```python
from build123d import *

# Parameters (mm, degrees)
ESQUISSE2_R             = 1.55
BOSS_EXTRU_1_DEPTH      = 6
ESQUISSE3_W             = 170
ESQUISSE3_H             = 35
ENL_V_MAT_EXTRU_1_DEPTH = 10
ENL_V_MAT_EXTRU_2_DEPTH = 2


with BuildPart() as part:
    # Esquisse2 → Boss.-Extru.1 (new body)
    with BuildSketch(Plane(origin=(0, 0, 0), x_dir=(1, 0, 0), z_dir=(0, 1, 0))):
        Polygon((30, 7.5), (-90, 7.5), (-100, 7.5), (-100, -7.5), (-90, -7.5), (30, -7.5), (40, -7.5), (50, -7.5), (50, 7.5), (40, 7.5), align=None)
        with Locations(Location((-90, 0, 0), (0, 0, 270))):
            Circle(ESQUISSE2_R, mode=Mode.SUBTRACT)
        with Locations(Location((0, 0, 0), (0, 0, 270))):
            Circle(ESQUISSE2_R, mode=Mode.SUBTRACT)
        with Locations(Location((40, 0, 0), (0, 0, 270))):
            Circle(ESQUISSE2_R, mode=Mode.SUBTRACT)
    extrude(amount=BOSS_EXTRU_1_DEPTH)

    # Esquisse3 → Enlèv. mat.-Extru.1 (cut)
    with BuildSketch(Plane.XZ):
        with Locations((-25, 0)):
            Rectangle(ESQUISSE3_W, ESQUISSE3_H)
        with BuildLine():
            Line((-90, -7.5), (-83.140864445, -7.5))
            Line((-83.140864445, -7.5), (-80, -5))
            Line((-80, -5), (0, -5))
            Line((0, -5), (30, -5))
            Line((30, -5), (33.140864445, -7.5))
            Line((33.140864445, -7.5), (40, -7.5))
            add(Edge.make_bspline(
                [(40, -7.5), (44.292893219, -7.707106781), (50.707106781, 0), (44.292893219, 7.707106781), (40, 7.5)],
                knots=[0, 0, 0, 0, 0.5, 1, 1, 1, 1], degree=3))
            Line((40, 7.5), (33.140864445, 7.5))
            Line((33.140864445, 7.5), (30, 5))
            Line((30, 5), (0, 5))
            Line((0, 5), (-80, 5))
            Line((-80, 5), (-83.140864445, 7.5))
            Line((-83.140864445, 7.5), (-90, 7.5))
            add(Edge.make_bspline(
                [(-90, -7.5), (-94.266151252, -7.718988485), (-100.733567708, 6.0631e-05), (-94.266713321, 7.718514748), (-90, 7.5)],
                knots=[0, 0, 0, 0, 0.500005708, 1, 1, 1, 1], degree=3))
        make_face(mode=Mode.SUBTRACT)
    extrude(amount=-ENL_V_MAT_EXTRU_1_DEPTH, mode=Mode.SUBTRACT)

    # Esquisse4 → Enlèv. mat.-Extru.2 (cut)
    with BuildSketch(Plane(origin=(0, 6, 0), x_dir=(1, 0, 0), z_dir=(0, 1, 0))):
        Polygon((-81.8, 3), (-80.7, 0), (-81.8, -3), (-8.2, -3), (-9.3, 0), (-8.2, 3), align=None)
    extrude(amount=-ENL_V_MAT_EXTRU_2_DEPTH, mode=Mode.SUBTRACT)


solid = part.part
```
Check sheet for the modelled part. Datum: model origin and axes. Units: mm. A direction names the side the tool comes from. Round coordinates to 2 decimals unless told otherwise and drop trailing zeros. Order: outer loops, then holes, each group sorted by start corner. A loop starts at its lowest first (then second) coordinate and runs counter-clockwise, first axis right, second up. Notation, with made-up numbers: (-33, 34.5) -> (23, 34.5) arc R13 ccw to (23, 41.5) -> close; hole circle Ø1 at (76, 67.25). An arc over 180 degrees is marked (long way). One line per item, written item: value. Start each with the question number.
Q1. Cross-section at A-A (x = 0). Record the boundary of the cut face in (y, z), and give its area (3 significant figures).
Q2. Mould release check, pull along X, two halves, no side actions. Record for faces 1 (the face through (-81.548, 2.958, 6.232)), 2 (the face through (-87, 3, -7.5)): pulls with the +X half, pulls with the -X half, needs draft (parallel to the pull), parting line crosses it, or undercut.
Q3. Cross-section at B-B (x = -21.5). Record the boundary of the cut face in (y, z).
Q4. Gauge pin test, flat ends, axial feed: pin 1 Ø2 at (y, z) = (5, -5.5) entering from -X; pin 2 Ø2 at (x, y) = (-24, 2.5) entering from +Z; pin 3 Ø1 at (x, y) = (-39, 5.5) entering from -Z. Record the tip position at first contact, or that the pin passes through.
Q5. Thickness scan on line 1 (X direction, y = 1.3, z = 0); line 2 (X direction, y = 4.25, z = 0); line 3 (Z direction, x = -90, y = 4.1). Record the ranges inside material, lowest first.
Q6. Cross-section at C-C (y = 1). Give the number of separate pieces and of enclosed holes in the cut face, and give its area (3 significant figures).
Q7. Set-up check for faces 3 (the face through (-24, 3, 5)), 4 (the face through (-46, 4, 0)), 5 (the face through (31.548, 2.958, -6.232)): record each of +Z, -Z, +X, -X, +Y, -Y from which the full face is reachable in a straight line by a thin tool's end or side.
Completed:
1. outline: (0, -5) -> (6, -5) -> (6, -1.55) -> (0, -1.55) -> close; (0, 1.55) -> (6, 1.55) -> (6, 5) -> (0, 5) -> close
1. area: 41.4 mm²
2. face 1: undercut
2. face 2: needs draft
3. outline: (0, -5) -> (6, -5) -> (6, -3) -> (4, -3) -> (4, 3) -> (6, 3) -> (6, 5) -> (0, 5) -> close
4. pin 1: stops at x = -96
4. pin 2: stops at z = 5
4. pin 3: stops at z = -5
5. line 1: x = -97.5 to -91.55, -88.45 to -1.55, 1.55 to 38.45, 41.55 to 47.5
5. line 2: x = -97.5 to -91.55, -88.45 to -80.7, -9.3 to -1.55, 1.55 to 38.45, 41.55 to 47.5
5. line 3: z = -7.5 to -1.55, 1.55 to 7.5
6. separate pieces: 1
6. enclosed holes: 3
6. area: 1,540 mm²
7. face 3: +Z, +Y, -Y
7. face 4: +Y
7. face 5: -Z, +Y, -Y
